Part model, mm, in its own coordinate system. Face numbers are marked on the shaded views. Coordinates: 2 decimals unless noted, no trailing zeros. Order: outer loops, then holes, each group sorted by start corner. A loop starts at its lowest first (then second) coordinate and runs counter-clockwise, first axis right, second up. Notation, with made-up numbers: (21.25, 13.5) - (35.25, 13.5) arc R28 cw to (35.25, 42.5) - close; hole circle Ø9 at (84.5, 16). An arc over 180 degrees is marked (long way). Use a Markdown table: item, result. Add a question column.
1) Saw through at C-C on y = 3.5. List the corners of the cut face in (x, z), then the cut area to 3 significant figures.
2) Two-plate mould, pull along Y, no slides. Class the marked faces 1, 2 and 3: +Y half, -Y half, draft (parallel to the pull), parting line (faces both ways), or undercut.
3) Saw through at A-A on y = 0. List the corners of the cut face in (x, z), then the cut area to 3 significant figures.
4) Saw through at D-D on z = 8.5. List the corners of the cut face in (x, y).
5) Drop flat-ended pins along their axis: P1, Ø3, axis at y = -2, z = 1, coming from the -X side; P2, Ø2.5, axis at x = 0, y = 0, coming from the -Z side; P3, Ø1.5, axis at y = -16.5, z = 8, coming from the +X side. Give the stop position or say it passes through.
6) Wall check: L1, parallel to Y at x = 0, z = 2.2; L2, parallel to Y at x = 0, z = 7.65; L3, parallel to X at y = -2, z = 7.5. Give the ranges that are in metal, low to high. Write a range as [from, to].
7) Saw through at B-B on z = 2.5. List the corners of the cut face in (x, y).
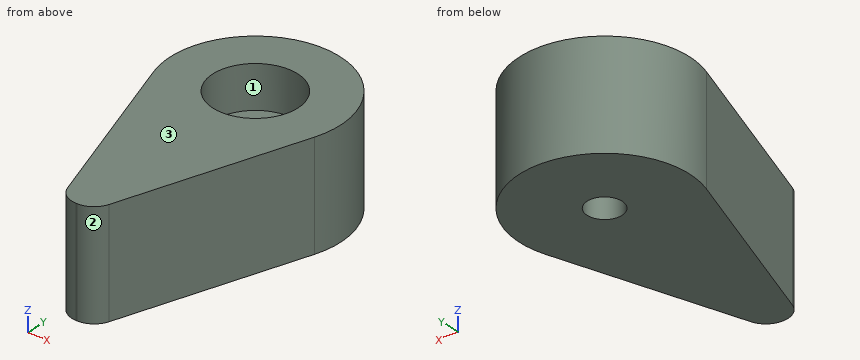
```python
from build123d import *

# Parameters (mm, degrees)
EXTRUDE_1_DEPTH     = 10
FILLET_1_R          = 2
SKETCH_4_R          = 4
CUT_EXTRUDE_1_DEPTH = 4
M4X0_71_D           = 3.3


with BuildPart() as part:
    # Эскиз1 → Бобышка-Вытянуть1 (new body)
    with BuildSketch(Plane.XY):
        with BuildLine():
            Line((-1.5, -21), (-7.597720185, -2.504924749))
            ThreePointArc((-7.597720185, -2.504924749), (0, 8), (7.597720185, -2.504924749))
            Line((7.597720185, -2.504924749), (1.5, -21))
            Line((1.5, -21), (-1.5, -21))
        make_face()
    extrude(amount=EXTRUDE_1_DEPTH)

    # Скругление1
    fillet_1_edges = [part.edges().sort_by_distance(p)[0] for p in [
        (-1.5, -21, 5),
        (1.5, -21, 5),
    ]]
    fillet(fillet_1_edges, radius=FILLET_1_R)

    # Эскиз4 → Вырез-Вытянуть1 (cut)
    with BuildSketch(Plane.XY.offset(10)):
        Circle(SKETCH_4_R)
    extrude(amount=-CUT_EXTRUDE_1_DEPTH, mode=Mode.SUBTRACT)

    # Отверстие обработанное метчиком M4x0.71 (through all)
    with Locations(Plane.XY.offset(6)):
        with Locations((0, 0)):
            Hole(M4X0_71_D / 2)


solid = part.part
```
Results are:
| question | item | result |
|---|---|---|
| 1 | outline | (-7.19, 0) - (7.19, 0) - (7.19, 10) - (1.94, 10) - (1.94, 6) - (-1.94, 6) - (-1.94, 10) - (-7.19, 10) - close |
| 1 | area | 128 mm2 |
| 2 | face 1 | undercut |
| 2 | face 2 | -Y half |
| 2 | face 3 | draft |
| 3 | outline | (-8, 0) - (-1.65, 0) - (-1.65, 6) - (-4, 6) - (-4, 10) - (-8, 10) - close; (1.65, 0) - (8, 0) - (8, 10) - (4, 10) - (4, 6) - (1.65, 6) - close |
| 3 | area | 108 mm2 |
| 4 | outline | (-7.6, -2.5) - (-1.95, -19.63) arc R2 ccw to (-0.05, -21) - (0.05, -21) arc R2 ccw to (1.95, -19.63) - (7.6, -2.5) arc R8 ccw (long way) to start; hole circle Ø8 at (0, 0) |
| 5 | P1 | x = -7.98 |
| 5 | P2 | through |
| 5 | P3 | x = 3.23 |
| 6 | L1 | [-21, -1.65], [1.65, 8] |
| 6 | L2 | [-21, -4], [4, 8] |
| 6 | L3 | [-7.75, -3.46], [3.46, 7.75] |
| 7 | outline | (-7.6, -2.5) - (-1.95, -19.63) arc R2 ccw to (-0.05, -21) - (0.05, -21) arc R2 ccw to (1.95, -19.63) - (7.6, -2.5) arc R8 ccw (long way) to start; hole circle Ø3.3 at (0, 0) |
